```python
from build123d import *

# Parameters (mm, degrees)
F0_R          = 1.5
F1_DEPTH      = 8
F1_DEPTH_BACK = 8
F2_DEPTH      = 6
F2_DEPTH_BACK = 6
F4_DEPTH      = 25


with BuildPart() as f1:
    # F0 (on Right) → F1 (new body, two sides)
    with BuildSketch(Plane.YZ) as f1_sk:
        with BuildLine():
            Line((-3, -10), (3, -10))
            Line((3, -10), (3, -7.486621))
            Line((3, -7.486621), (3, 7))
            ThreePointArc((3, 7), (2.12132, 9.12132), (0, 10))
            ThreePointArc((0, 10), (-2.12132, 9.12132), (-3, 7))
            Line((-3, 7), (-3, -7.486621))
            Line((-3, -7.486621), (-3, -10))
        make_face()
        with Locations((0, 7)):
            Circle(F0_R, mode=Mode.SUBTRACT)
    extrude(amount=F1_DEPTH)
    extrude(f1_sk.sketch, amount=-F1_DEPTH_BACK)

    # F0 (on Right) → F2 (join, two sides)
    with BuildSketch(Plane.YZ) as f2_sk:
        with BuildLine():
            Line((3, 7), (3, -7.486621))
            Line((3, -7.486621), (4.5, -7.486621))
            Line((4.5, -7.486621), (4.5, 7))
            ThreePointArc((4.5, 7), (3.181981, 10.181981), (0, 11.5))
            ThreePointArc((0, 11.5), (-3.181981, 10.181981), (-4.5, 7))
            Line((-4.5, 7), (-4.5, -7.486621))
            Line((-4.5, -7.486621), (-3, -7.486621))
            Line((-3, -7.486621), (-3, 7))
            ThreePointArc((-3, 7), (-2.12132, 9.12132), (0, 10))
            ThreePointArc((0, 10), (2.12132, 9.12132), (3, 7))
        make_face()
    extrude(amount=F2_DEPTH)
    extrude(f2_sk.sketch, amount=-F2_DEPTH_BACK)

    # F3 (on face) → F4 (cut)
    with BuildSketch(Plane.XZ.offset(4.5)):
        with BuildLine():
            Line((2, -3), (2, 3))
            ThreePointArc((2, 3), (1.414214, 4.414214), (0, 5))
            ThreePointArc((0, 5), (-1.414214, 4.414214), (-2, 3))
            Line((-2, 3), (-2, -3))
            ThreePointArc((-2, -3), (-1.414214, -4.414214), (0, -5))
            ThreePointArc((0, -5), (1.414214, -4.414214), (2, -3))
        make_face()
    extrude(amount=-F4_DEPTH, mode=Mode.SUBTRACT)


solid = f1.part
```
The model under review builds one solid part; all positions refer to its coordinate system, in mm. A direction names the side the tool comes from. Round coordinates to 2 decimals unless told otherwise and drop trailing zeros. Write each loop counter-clockwise with the first axis right and the second up, starting at its lowest first coordinate (ties: lowest second). Pieces come first, ordered by that corner, then holes.
(1) Mouldability with a two-part tool opening along X and no side actions: class faces 6 (the flat face through (-1, 3, -8)), 7 (the flat face through (-8, 0, 0)), 8 (the flat face through (-2, 0, 0)) as +X half, -X half, draft (parallel to the pull), parting line (faces both ways), or undercut.
(2) We need section D-D on y = 2.5. Give the boundary of the cut face in (x, z), and give its area (3 significant figures).
(3) We need section B-B on x = 2.75. Give the boundary of the cut face in (y, z).
(4) We need section A-A on z = 0. Give the boundary of the cut face in (x, y).
(5) Machinability: for faces 1 (the flat face through (6, -4, 2)), 2 (the flat face through (2, 0, 0)), 3 (the flat face through (0, -4, -7.487)), 4 (the flat face through (-6, -4, 2)), 5 (the flat face through (0, 4, -7.487)), which of the approach directions +Z, -Z, +X, -X, +Y, -Y give a long, thin tool a straight path to every point of the face, cutting with its end or side? Answer none if there is none.
(6) We need section C-C on y = 0.25. Give the boundary of the cut face in (x, z).
(7) Insertion check: pin 1 (0.8 mm diameter, centred on x = -2, y = 4, fed in from -Z); pin 2 (1.5 mm diameter, centred on x = -6, y = -1.5, fed in from +Z). Each pin has a flat end and moves straight along its axis. Give the tip position at first contact, or say it passes through.
(8) Wall thickness on L1, parallel to X at y = 2.25, z = -2.25; L2, parallel to Z at x = 0.25, y = -0.25; L3, parallel to X at y = 4, z = -2.5: over which ranges is each line inside the solid? List them lowest first.
Findings below:
1. face 6: draft
1. face 7: -X half
1. face 8: undercut
2. outline: (-8, -10) - (8, -10) - (8, 8.66) - (6, 8.66) - (6, 10.74) - (-6, 10.74) - (-6, 8.66) - (-8, 8.66) - close; hole (-2, -3) arc R2 ccw to (0, -5) arc R2 ccw to (2, -3) - (2, 3) arc R2 ccw to (0, 5) arc R2 ccw to (-2, 3) - close
2. area: 287 mm2
3. outline: (-4.5, -7.49) - (-3, -7.49) - (-3, -10) - (3, -10) - (3, -7.49) - (4.5, -7.49) - (4.5, 7) arc R4.5 ccw to (0, 11.5) arc R4.5 ccw to (-4.5, 7) - close; hole circle Ø3 at (0, 7)
4. outline: (-8, -3) - (-6, -3) - (-6, -4.5) - (-2, -4.5) - (-2, 4.5) - (-6, 4.5) - (-6, 3) - (-8, 3) - close; (2, -4.5) - (6, -4.5) - (6, -3) - (8, -3) - (8, 3) - (6, 3) - (6, 4.5) - (2, 4.5) - close
5. face 1: +Z, +X
5. face 2: +Y, -Y
5. face 3: -Z, +X, -X, -Y
5. face 4: +Z, -X
5. face 5: -Z, +X, -X, +Y
6. outline: (-8, -10) - (8, -10) - (8, 5.52) - (-8, 5.52) - close; (-8, 8.48) - (8, 8.48) - (8, 9.99) - (6, 9.99) - (6, 11.49) - (-6, 11.49) - (-6, 9.99) - (-8, 9.99) - close; hole (-2, -3) arc R2 ccw to (0, -5) arc R2 ccw to (2, -3) - (2, 3) arc R2 ccw to (0, 5) arc R2 ccw to (-2, 3) - close
7. pin 1: stops at z = -7.49
7. pin 2: stops at z = 11.44
8. L1: x = -8 to -2, 2 to 8
8. L2: z = -10 to -4.98, 4.98 to 5.52, 8.48 to 11.49
8. L3: x = -6 to -2, 2 to 6
